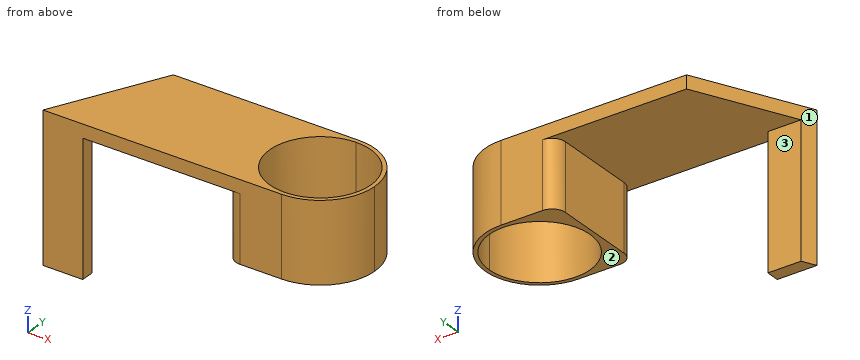
from build123d import *

# Parameters (mm, degrees)
F1_DEPTH = 55
F3_DEPTH = 50
F4_W     = 46.665443
F4_H     = 57.836632
F5_DEPTH = 25
F6_R     = 5


with BuildPart() as f1:
    # F0 (on Top) → F1 (new body)
    with BuildSketch(Plane.XY):
        with BuildLine():
            ThreePointArc((19, 0), (13.435029, 13.435029), (0, 19))
            ThreePointArc((0, 19), (-13.435029, -13.435029), (19, 0))
        make_face()
        with BuildLine():
            ThreePointArc((0, -20.5), (14.495689, -14.495689), (20.5, 0))
            ThreePointArc((20.5, 0), (14.495689, 14.495689), (0, 20.5))
            ThreePointArc((0, 20.5), (-20.5, 0), (0, -20.5))
        make_face()
        with BuildLine():
            ThreePointArc((19, 0), (-13.435029, -13.435029), (0, 19))
            ThreePointArc((0, 19), (13.435029, 13.435029), (19, 0))
        make_face(mode=Mode.SUBTRACT)
        with BuildLine():
            ThreePointArc((0, -20.5), (-20.5, 0), (0, 20.5))
            Line((0, 20.5), (-70, 20.5))
            Line((-70, 20.5), (-90, -20.5))
            Line((-90, -20.5), (0, -20.5))
        make_face()
    extrude(amount=F1_DEPTH)

    # F2 (on face) → F3 (cut)
    with BuildSketch(Plane.XY):
        Polygon((-20.693906, 24.132871), (-92.302133, 24.132871), (-92.683225, -15.5), (-75, -15.5), (-75, -22.003565), (-20.745235, -22.003565), align=None)
    extrude(amount=F3_DEPTH, mode=Mode.SUBTRACT)

    # F4 (on face) → F5 (cut)
    with BuildSketch(Plane.XY):
        with Locations((-0.75581, 1.738093)):
            Rectangle(F4_W, F4_H)
    extrude(amount=F5_DEPTH, mode=Mode.SUBTRACT)

    # F6
    f6_edges = [f1.edges().sort_by_distance(p)[0] for p in [
        (-20.697947, 20.5, 37.5),
        (-20.743562, -20.5, 37.5),
    ]]
    fillet(f6_edges, radius=F6_R)


solid = f1.part
Here's how the part is built. I have some questions about the finished solid (model axes, mm). Face numbers are marked on the shaded views. A direction names the side the tool comes from. Coordinates: 2 decimals unless noted, no trailing zeros. Write each loop counter-clockwise with the first axis right and the second up, starting at its lowest first coordinate (ties: lowest second). Pieces come first, ordered by that corner, then holes.
Item 1: I want a section at A-A on z = 42.5. Write out the boundary of the cut face in (x, y).
Item 2: If I drill on line 1 (X direction, y = 0, z = 48); line 2 (Z direction, x = -33, y = 5.5); line 3 (X direction, y = 8.5, z = 34), over which ranges is the centre line in solid material (lowest first)?
Item 3: On a 3-axis mill with a long thin cutter (end or side, diameter ignored), from which of +Z, -Z, +X, -X, +Y, -Y can I reach the whole of each face in a straight line? I mean the marked faces 1, 2 and 3. Say none if no direction works.
Item 4: I want a section at D-D on x = -43.5. Write out the boundary of the cut face in (y, z), and give its area (3 significant figures).
Item 5: I want a section at B-B on y = 6. Write out the boundary of the cut face in (x, z), and give its area (3 significant figures).
Item 6: I want a section at C-C on x = 8.5. Write out the boundary of the cut face in (y, z).
Item 7: Will these pins go through, and if not, where does the flat tip stop? pin 1 (2.5 mm diameter, centred on y = -17, z = 29.5, fed in from +X); pin 2 (10 mm diameter, centred on x = -49.5, y = -0.5, fed in from -Z); pin 3 (1.5 mm diameter, centred on x = -74.5, z = 34, fed in from +Y).
Findings below:
1. outline: (-90, -20.5) - (-75, -20.5) - (-75, -15.5) - (-87.56, -15.5) - close; (-20.74, -15.49) arc R5 ccw to (-15.74, -20.5) - (0, -20.5) arc R20.5 ccw to (0, 20.5) - (-15.7, 20.5) arc R5 ccw to (-20.7, 15.51) - close; hole circle Ø38 at (0, 0)
2. line 1: x = -20.72 to -19, 19 to 20.5
2. line 2: z = 50 to 55
2. line 3: x = -20.71 to -16.99, 16.99 to 18.65
3. face 1: +Z, -Z, -X, +Y
3. face 2: -Z, +X, +Y, -Y
3. face 3: -Z, -X, +Y
4. outline: (-20.5, 50) - (20.5, 50) - (20.5, 55) - (-20.5, 55) - close
4. area: 205 mm2
5. outline: (-77.07, 50) - (-20.71, 50) - (-20.71, 25) - (-18.03, 25) - (-18.03, 55) - (-77.07, 55) - close; (18.03, 25) - (19.6, 25) - (19.6, 55) - (18.03, 55) - close
5. area: 410 mm2
6. outline: (-18.65, 25) - (-16.99, 25) - (-16.99, 55) - (-18.65, 55) - close; (16.99, 25) - (18.65, 25) - (18.65, 55) - (16.99, 55) - close
7. pin 1: stops at x = 13.12
7. pin 2: stops at z = 50
7. pin 3: stops at y = -15.5
